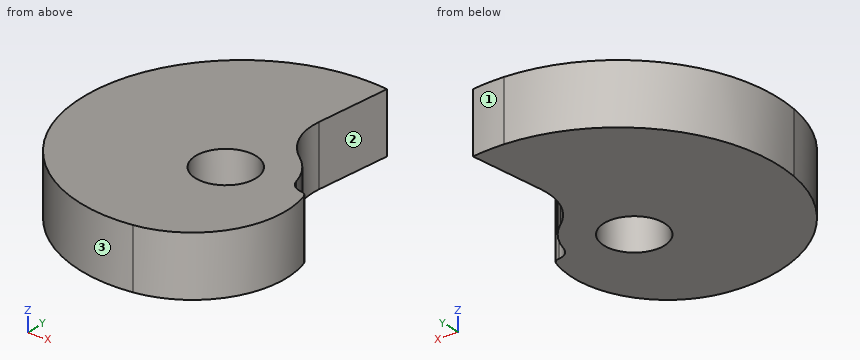
Autodesk Inventor part; units mm, degrees
ref_plane "YZ Plane" through (0, 0, 0) normal (1, 0, 0) x (0, 1, 0)
ref_plane "XZ Plane" through (0, 0, 0) normal (0, 1, 0) x (-1, 0, 0)
ref_plane "XY Plane" through (0, 0, 0) normal (0, 0, 1) x (1, 0, 0)
sketch "Sketch1" plane through (0, 0, 0) normal (0, 0, 1) x (1, 0, 0)
  circle A0 centre (0, 0) radius 3.175
  circle A1 centre (0, 0) radius 19.05
  circle A2 centre (40.4812, 19.05) radius 38.1 construction
  line L0 (2.3815, 18.9005) -> (40.4812, 19.05) construction
  circle A3 centre (0, 0) radius 6.35
  circle A4 centre (0, 0) radius 7.9375 construction
  line L1 (0, 0) -> (2.3815, 18.9005)
  line L2 (0, 0) -> (-0.9367, 19.027) construction
  line L3 (40.4812, 19.05) -> (6.35, 0) construction
  line L4 (0, 0) -> (7.9375, 0) construction
  circle A5 centre (0, 0) radius 12.7 construction
  circle A6 centre (0, 0) radius 16.6688 construction
  arc A7 (0, -12.7) -> (7.8908, 0.86) centre (-1.2714, -2.8843) ccw
  line L5 (0, 0) -> (0, -12.7) construction
  line L6 (0, 0) -> (-19.05, 0) construction
  arc A8 (-16.6688, 0) -> (0, -12.7) centre (-1.914, 2.0767) ccw
  arc A9 (-0.9367, 19.027) -> (-16.6688, 0) centre (-0.1147, 2.33) ccw
  circle A10 centre (7.682, 1.9978) radius 1.5875
  line L7 (7.8908, 0.86) -> (9.2192, 1.6014)
  point P0 (0.7938, 6.3002)
  point P1 (7.2124, 0.4813)
  point P2 (6.1456, 1.5983)
  point P3 (8.0468, 0.4528)
  dimension "d5" = 12.7
  dimension "d15" = 25.4
  dimension "d16" = 33.3375
  dimension "d0" = 6.35
  dimension "d1" = 38.1
  dimension "d2" = 76.2
  dimension "d6" = 15.875
  dimension "d11" = 19.05
  dimension "d12" = 40.4813
  dimension "d13" = 10
  dimension "d14" = 28.943
  dimension "d20" = 3.175
extrude "Extrusion1" add sketch "Sketch1" along normal blind 6.35 contours A3 | A3 A10 A7 A8 A9 A1 L1 picked at (-2.1715, 14.5665)
fillet "Fillet1" radius 6.35 1 edges at (0.7938, 6.3002, 3.175)
fillet "Fillet3" radius 0.7937 1 edges at (8.0468, 0.4528, 3.175)
properties part number "Snail V2" material "UHMW, White"
Design review of the part built by this model. Coordinates are the model's own, in mm. Face numbers are marked on the shaded views. Give positions to 0.01 mm unless a question says otherwise; leave off trailing zeros. Loops run counter-clockwise (first coordinate to the right, second up) from the corner with the lowest first, then second, coordinate; pieces in that order, holes last. Notation, with made-up numbers: (17.5, 53.25) - (56.5, 53.25) arc R22 ccw to (56.5, 71.25) - close; hole circle Ø9 at (43, 87.25). An arc over 180 degrees is marked (long way). Use CSV: the item, a comma, the result in double quotes. Start each with the question number.
1. Add section C-C (y = 6). State the section outline as (x, z) points.
2. Wall thickness on L1, parallel to Y at x = 0, z = 4.5 (3 decimals); L2, parallel to X at y = 0, z = 1.5 (3 decimals); L3, parallel to X at y = -2, z = 3.25: over which ranges is each line inside the solid? List them lowest first.
3. Add section A-A (y = -2). State the section outline as (x, z) points.
4. Draft analysis for pull direction Y (two halves, no side actions). For the marked faces 1, 2 and 3, state which applies: released by +Y, released by -Y, zero draft, split by the parting line, or undercut.
5. Insertion check: P1, Ø5, axis at x = 0, y = 0, coming from the -Z side; P2, Ø3, axis at y = -8, z = 1, coming from the -X side; P3, Ø1.5, axis at y = -9, z = 1.5, coming from the -X side. Each pin has a flat end and moves straight along its axis. Give the tip position at first contact, or say it passes through.
6. Add section B-B (x = -9). State the section outline as (y, z) points.
Results found:
1,outline,"(-16.42, 0) - (2.84, 0) - (2.84, 6.35) - (-16.42, 6.35) - close"
2,L1,"y = -12.7 to -3.175, 3.175 to 19.05"
2,L2,"x = -16.669 to -3.175, 3.175 to 8.18"
2,L3,"x = -16.25 to -2.47, 2.47 to 8.59"
3,outline,"(-16.25, 0) - (-2.47, 0) - (-2.47, 6.35) - (-16.25, 6.35) - close; (2.47, 0) - (8.59, 0) - (8.59, 6.35) - (2.47, 6.35) - close"
4,face 1,"released by +Y"
4,face 2,"undercut"
4,face 3,"released by -Y"
5,P1,"passes through"
5,P2,"stops at x = -14.1"
5,P3,"stops at x = -12.66"
6,outline,"(-11.03, 0) - (16.49, 0) - (16.49, 6.35) - (-11.03, 6.35) - close"
